Can you work these out from the model? Positions are in its coordinate system, mm. A direction names the side the tool comes from. Give positions to 0.01 mm unless a question says otherwise; leave off trailing zeros. Order: outer loops, then holes, each group sorted by start corner. A loop starts at its lowest first (then second) coordinate and runs counter-clockwise, first axis right, second up. Notation, with made-up numbers: (46, -24.75) -> (65, -24.75) arc R28 cw to (65, 1.25) -> close; hole circle Ø7 at (-20, 60.5). An arc over 180 degrees is marked (long way). Answer as CSV lines item,"result".
Autodesk Inventor part; units mm, degrees
ref_plane "YZ Plane" through (0, 0, 0) normal (1, 0, 0) x (0, 1, 0)
ref_plane "XZ Plane" through (0, 0, 0) normal (0, 1, 0) x (-1, 0, 0)
ref_plane "XY Plane" through (0, 0, 0) normal (0, 0, 1) x (1, 0, 0)
sketch "Sketch1" plane through (0, 0, 0) normal (0, 0, 1) x (1, 0, 0)
  line L0 (-16.8, 0) -> (2.8, 0) construction
  line L1 (0, -0.5) -> (0, 3) construction
  line L2 (0, 0) -> (0, 1.1726)
  line L3 (-1, 2.5) -> (-14, 2.5)
  line L4 (-14, 2.5) -> (-14, 1.75)
  line L5 (-14, 1.75) -> (-3, 1.75)
  line L6 (-3, 1.75) -> (-3, 0)
  line L7 (-3, 0) -> (0, 0)
  line L8 (-1, 2.5) -> (-1, 1.75)
  line L9 (-1, 1.75) -> (0, 1.1726)
  dimension "d0" = 5
  dimension "d1" = 3.5
  dimension "d3" = 14
  dimension "d6" = 2
  dimension "d7" = 60
  dimension "d9" = 1
revolve "Revolution1" add sketch "Sketch1" angle 360 about axis through (-10, 0, 0) along (1, 0, 0)
fillet "Fillet2" radius 1 1 edges at (-1, -2.5, 0)
properties part number "P110" material "ABS Plastic"
Item 1: For pin 1 (1.5 mm diameter, centred on x = -6, z = 2, fed in from +Y); pin 2 (1.5 mm diameter, centred on x = -7, y = 2, fed in from +Z); pin 3 (1 mm diameter, centred on x = -2.5, z = 0.5, fed in from -Y), each with a flat end and sliding along its axis, tell me the tip position at first contact or that it passes through.
Numbers:
pin 1,"stops at y = 2.17"
pin 2,"stops at z = 2.17"
pin 3,"stops at y = -2.5"
Item 2: We'd pull the mould along Y, two halves only. Please class faces 1 (the cylindrical face through (-8.07, -0.54, 2.44)), 2 (the cylindrical face through (-8.423, 1.617, -0.67)), 3 (the flat face through (0, 0, 0)): released by +Y, released by -Y, zero draft, split by the parting line, or undercut.
Numbers:
face 1,"split by the parting line"
face 2,"undercut"
face 3,"zero draft"
Item 3: For faces 4 (the flat face through (-3, 0, 0)), 5 (the flat face through (-14, 1, 2)), which set-ups out of +Z, -Z, +X, -X, +Y, -Y let a thin tool reach every point of the face, with its end or its side?
Numbers:
face 4,"-X"
face 5,"+Z, -Z, -X, +Y, -Y"
Item 4: Please list where these lines run through material, in increasing order: line 1 along Z through (x, y) = (-7.5, 0); line 2 along Z through (x, y) = (-5.25, -1.2); line 3 along Y through (x, z) = (-12.25, -0.8).
Numbers:
line 1,"z = -2.5 to -1.75, 1.75 to 2.5"
line 2,"z = -2.19 to -1.27, 1.27 to 2.19"
line 3,"y = -2.37 to -1.56, 1.56 to 2.37"
Item 5: Imagine slicing it at C-C, the plane x = -3.5. Please give me the cut outline in (y, z).
Numbers:
outline,"circle Ø5 at (0, 0); hole circle Ø3.5 at (0, 0)"
Item 6: Imagine slicing it at A-A, the plane z = 0. Please give me the cut outline in (x, y).
Numbers:
outline,"(-14, -2.5) -> (-1.97, -2.5) arc R1 ccw to (-1, -1.75) -> (0, -1.17) -> (0, 1.17) -> (-1, 1.75) arc R1 ccw to (-1.97, 2.5) -> (-14, 2.5) -> (-14, 1.75) -> (-3, 1.75) -> (-3, -1.75) -> (-14, -1.75) -> close"
